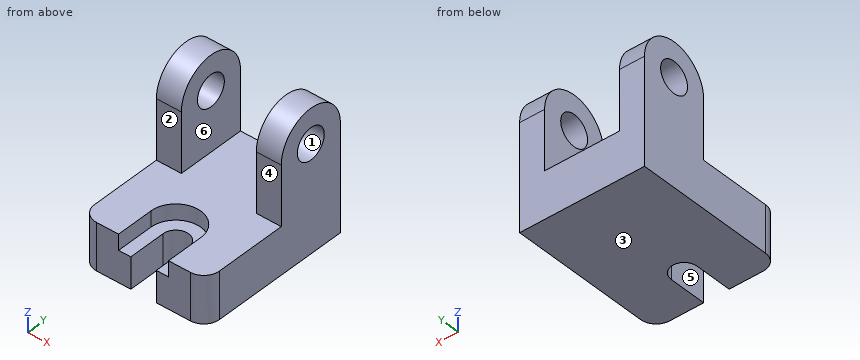
from build123d import *

# Parameters (mm, degrees)
F0_R     = 10
F1_DEPTH = 40
F2_DEPTH = 24
F3_W     = 7.84
F3_H     = 5
F3_W_2   = 16.32
F4_DEPTH = 10
F3_H_2   = 24
F5_DEPTH = 30
F6_R     = 10


with BuildPart() as f1:
    # F0 (on Right) → F1 (new body, symmetric)
    with BuildSketch(Plane.YZ):
        Polygon((0, 30), (0, 0), (100, 0), (100, 30), (56, 30), align=None)
        with BuildLine():
            Line((56, 68), (56, 30))
            Line((56, 30), (100, 30))
            Line((100, 30), (100, 68))
            ThreePointArc((100, 68), (78, 46), (56, 68))
        make_face()
        with BuildLine():
            ThreePointArc((100, 68), (78, 90), (56, 68))
            ThreePointArc((56, 68), (78, 46), (100, 68))
        make_face()
        with Locations((78, 68)):
            Circle(F0_R, mode=Mode.SUBTRACT)
    extrude(amount=F1_DEPTH, both=True)

    # F0 (on Right) → F2 (cut, symmetric)
    with BuildSketch(Plane.YZ):
        with BuildLine():
            Line((56, 68), (56, 30))
            Line((56, 30), (100, 30))
            Line((100, 30), (100, 68))
            ThreePointArc((100, 68), (78, 46), (56, 68))
        make_face()
        with BuildLine():
            ThreePointArc((100, 68), (78, 90), (56, 68))
            ThreePointArc((56, 68), (78, 46), (100, 68))
        make_face()
        with Locations((78, 68)):
            Circle(F0_R, mode=Mode.SUBTRACT)
    extrude(amount=F2_DEPTH, both=True, mode=Mode.SUBTRACT)

    # F3 (on face) → F4 (cut)
    with BuildSketch(Plane.XY.offset(30)):
        with Locations((-12.08, 2.5)):
            Rectangle(F3_W, F3_H)
        with BuildLine():
            Line((-16, 24), (-16, 5))
            Line((-16, 5), (-8.16, 5))
            Line((-8.16, 5), (-8.16, 24))
            ThreePointArc((-8.16, 24), (0, 32.16), (8.16, 24))
            Line((8.16, 24), (8.16, 5))
            Line((8.16, 5), (16, 5))
            Line((16, 5), (16, 24))
            ThreePointArc((16, 24), (0, 40), (-16, 24))
        make_face()
        with Locations((12.08, 2.5)):
            Rectangle(F3_W, F3_H)
        with Locations((0, 2.5)):
            Rectangle(F3_W_2, F3_H)
        with BuildLine():
            Line((-8.16, 24), (-8.16, 5))
            Line((-8.16, 5), (8.16, 5))
            Line((8.16, 5), (8.16, 24))
            ThreePointArc((8.16, 24), (0, 32.16), (-8.16, 24))
        make_face()
    extrude(amount=-F4_DEPTH, mode=Mode.SUBTRACT)

    # F3 (on face) → F5 (cut, through all)
    with BuildSketch(Plane.XY.offset(30)):
        with BuildLine():
            Line((-8.16, 24), (-8.16, 5))
            Line((-8.16, 5), (8.16, 5))
            Line((8.16, 5), (8.16, 24))
            ThreePointArc((8.16, 24), (0, 32.16), (-8.16, 24))
        make_face()
        with Locations((0, 2.5)):
            Rectangle(F3_W_2, F3_H)
        with Locations((0, -12)):
            Rectangle(F3_W_2, F3_H_2)
    extrude(amount=-F5_DEPTH, mode=Mode.SUBTRACT)

    # F6
    f6_edges = [f1.edges().sort_by_distance(p)[0] for p in [
        (-40, 0, 15),
        (40, 0, 15),
    ]]
    fillet(f6_edges, radius=F6_R)


solid = f1.part
Can you work these out from the model? Positions are in its coordinate system, mm. Face numbers are marked on the shaded views. A direction names the side the tool comes from. Coordinates: 2 decimals unless noted, no trailing zeros. Write each loop counter-clockwise with the first axis right and the second up, starting at its lowest first coordinate (ties: lowest second). Pieces come first, ordered by that corner, then holes. Notation, with made-up numbers: (33.5, 31) - (76.5, 31) arc R31 cw to (76.5, 56) - close; hole circle Ø11 at (61.5, -37.5). An arc over 180 degrees is marked (long way). Return JSON: item names as keys, results as strings. Group by question number.
Item 1: We'd pull the mould along Z, two halves only. Please class the marked faces 1, 2 and 3: pulls with the +Z half, pulls with the -Z half, needs draft (parallel to the pull), parting line crosses it, or undercut.
Item 2: If we section it at A-A (x = -25.5): Write out the boundary of the cut face in (y, z).
Item 3: Please list where these lines run through material, in increasing order: probe 1 along X at (y, z) = (61, 56); probe 2 along Z at (x, y) = (-27.25, 78); probe 3 along Z at (x, y) = (23, 45.5).
Item 4: Which directions (+Z, -Z, +X, -X, +Y, -Y) give clear straight access to the entire face, cutting with the end or side of a thin tool? Please do the marked faces 4, 5 and 6.
Item 5: I'm going to push flat-ended pins straight in: pin 1 Ø3 at (y, z) = (7.5, 22.5) entering from -X; pin 2 Ø1.5 at (x, y) = (-23, 23.5) entering from +Z; pin 3 Ø13 at (x, z) = (-33, 57) entering from -Y. Where does each tip first touch, or does it pass through?
Item 6: If we section it at D-D (z = 17.5): Write out the boundary of the cut face in (x, y).
Item 7: If we section it at C-C (z = 44): Write out the boundary of the cut face in (x, y).
Item 8: If we section it at B-B (y = 78): Write out the boundary of the cut face in (x, z).
Return value:
{
 "1": {"face 1": "undercut", "face 2": "needs draft", "face 3": "pulls with the -Z half"},
 "2": {"outline": "(0, 0) - (100, 0) - (100, 68) arc R22 ccw to (56, 68) - (56, 30) - (0, 30) - close; hole circle Ø20 at (78, 68)"},
 "3": {"probe 1": "x = -40 to -24, 24 to 40", "probe 2": "z = 0 to 58, 78 to 90", "probe 3": "z = 0 to 30"},
 "4": {"face 4": "+Z, +X, -X, -Y", "face 5": "+Z, -Z, -Y", "face 6": "+Z, +Y, -Y"},
 "5": {"pin 1": "stops at x = -39.95", "pin 2": "stops at z = 30", "pin 3": "stops at y = 56"},
 "6": {"outline": "(-40, 10) arc R10 ccw to (-30, 0) - (-8.16, 0) - (-8.16, 24) arc R8.16 cw to (8.16, 24) - (8.16, 0) - (30, 0) arc R10 ccw to (40, 10) - (40, 100) - (-40, 100) - close"},
 "7": {"outline": "(-40, 56) - (-24, 56) - (-24, 100) - (-40, 100) - close; (24, 56) - (40, 56) - (40, 100) - (24, 100) - close"},
 "8": {"outline": "(-40, 0) - (40, 0) - (40, 58) - (24, 58) - (24, 30) - (-24, 30) - (-24, 58) - (-40, 58) - close; (-40, 78) - (-24, 78) - (-24, 90) - (-40, 90) - close; (24, 78) - (40, 78) - (40, 90) - (24, 90) - close"}
}
